```python
from build123d import *

# Parameters (mm, degrees)
F0_W      = 30
F0_H      = 30
F1_DEPTH  = 165
F3_DEPTH  = 30
F4_R      = 5.5
F5_DEPTH  = 12.3
F6_R      = 8
F6_R_2    = 6.5
F7_DEPTH  = 2
F8_SIZE   = 3
F10_DEPTH = 25


# Not quite as in the source:
# - a pattern or mirror of a feature is missing from the dataset's text; its kind, count and spacing are read off the source's solid


with BuildPart() as f1:
    # F0 (on Front) → F1 (new body)
    with BuildSketch(Plane.XZ):
        Rectangle(F0_W, F0_H)
    extrude(amount=F1_DEPTH)

    # F2 (on face) → F3 (cut)
    with BuildSketch(Plane.XY.offset(15)):
        with BuildLine():
            ThreePointArc((0, -8.5), (-4.5961940777, -19.5961940777), (6.5, -15))
            ThreePointArc((6.5, -15), (4.5961940777, -10.4038059223), (0, -8.5))
        make_face()
    extrude(amount=-F3_DEPTH, mode=Mode.SUBTRACT)

    # F4 (on face) → F5 (cut)
    with BuildSketch(Plane.YZ.offset(15)):
        with Locations((-15, 0)):
            Circle(F4_R)
    extrude(amount=-F5_DEPTH, mode=Mode.SUBTRACT)

    # F6 (on face) → F7 (cut)
    with BuildSketch(Plane.XY.offset(15)):
        with Locations((0, -15)):
            Circle(F6_R)
        with Locations((0, -15)):
            Circle(F6_R_2, mode=Mode.SUBTRACT)
        with Locations((0, -15)):
            Circle(F6_R_2)
    f7 = extrude(amount=-F7_DEPTH, mode=Mode.SUBTRACT)

    # F7_copies: F7 across plane
    add(f7.mirror(Plane(origin=(0, 0, 0), x_dir=(-1, 0, 0), z_dir=(0, 0, -1))), mode=Mode.SUBTRACT)

    # F8
    f8_edges = [f1.edges().sort_by_distance(p)[0] for p in [
        (15, -82.5, 15),
        (0, 0, 15),
        (-15, -82.5, 15),
        (0, -165, 15),
    ]]
    chamfer(f8_edges, length=F8_SIZE)

    # F9 (on face) → F10 (cut)
    with BuildSketch(Plane(origin=(0, 0, -15), x_dir=(1, 0, 0), z_dir=(0, 0, -1))):
        with BuildLine():
            ThreePointArc((0, 90.5), (-4, 86.5), (0, 82.5))
            Line((0, 82.5), (0, 86.5))
            Line((0, 86.5), (0, 90.5))
        make_face()
        with BuildLine():
            Line((0, 86.5), (0, 82.5))
            ThreePointArc((0, 82.5), (2.8284271247, 83.6715728753), (4, 86.5))
            ThreePointArc((4, 86.5), (2.8284271247, 89.3284271247), (0, 90.5))
            Line((0, 90.5), (0, 86.5))
        make_face()
        with BuildLine():
            ThreePointArc((4, 156.5), (-2.8284271247, 159.3284271247), (0, 152.5))
            ThreePointArc((0, 152.5), (2.8284271247, 153.6715728753), (4, 156.5))
        make_face()
    extrude(amount=-F10_DEPTH, mode=Mode.SUBTRACT)


solid = f1.part
```
Can you work these out from the model? Positions are in its coordinate system, mm. A direction names the side the tool comes from. Give positions to 0.01 mm unless a question says otherwise; leave off trailing zeros. Loops run counter-clockwise (first coordinate to the right, second up) from the corner with the lowest first, then second, coordinate; pieces in that order, holes last. Notation, with made-up numbers: M -33.75,-32 L 22.25,-32 A20 ccw 22.25,-27 Z; hole C 53,-35.5 d8. An arc over 180 degrees is marked long. One line per question, with ' | ' between items. Start each with the question number.
Q1. If we section it at B-B (z = -8.5): Please give me the cut outline in (x, y).
Q2. If we mould it in two halves opening along X, with no side actions, what happens to faces 1 (the flat face through (0, -164, 13)), 2 (the flat face through (-13, -81, 14)), 3 (the flat face through (0, -8, -13))? For each: +X half, -X half, draft (parallel to the pull), parting line (faces both ways), or undercut.
Q3. For pin 1 Ø2.5 at (x, y) = (-2, -88.5) entering from -Z; pin 2 Ø10.5 at (x, y) = (0, -15) entering from +Z, each with a flat end and sliding along its axis, tell me the tip position at first contact or that it passes through.
Q4. If I drill on line 1 (X direction, y = -156.5, z = 2.5); line 2 (Z direction, x = 7, y = -15); line 3 (X direction, y = -15, z = 5.75), over which ranges is the centre line in solid material (lowest first)? Write a range as from..to.
Q5. For faces 4 (the flat face through (0, -87, 10)), 5 (the cylindrical face through (10.595, -9.754, 1.652)), 6 (the cylindrical face through (7.63, -12.6, 14.01)), which set-ups out of +Z, -Z, +X, -X, +Y, -Y let a thin tool reach every point of the face, with its end or its side?
Q6. If we section it at A-A (z = 0): Please give me the cut outline in (x, y), plus the area to 3 significant figures.
Computed:
1) outline: M -15,-165 L 15,-165 L 15,0 L -15,0 Z; hole C 0,-15 d13; hole C 0,-156.5 d8; hole C 0,-86.5 d8
2) face 1: draft | face 2: -X half | face 3: undercut
3) pin 1: stops at z = -15 | pin 2: passes through
4) line 1: x = -15..-4, 4..15 | line 2: z = -13..-5.5, 5.5..13 | line 3: x = -15..-6.5, 6.5..15
5) face 4: -Z | face 5: +X | face 6: +Z
6) outline: M -15,-165 L 15,-165 L 15,-20.5 L 3.46,-20.5 A6.5 cw long 3.46,-9.5 L 15,-9.5 L 15,0 L -15,0 Z; hole C 0,-156.5 d8; hole C 0,-86.5 d8 | area: 4,610 mm²
